Design review of the part shown in the three views and the two pictorial views. Dimensions are in mm from the part's minimum x, y and z. Coordinates: 2 decimals unless noted, no trailing zeros. Loops run counter-clockwise (first coordinate to the right, second up) from the corner with the lowest first, then second, coordinate; pieces in that order, holes last. Notation, with made-up numbers: M -34.75,12 L 20.25,12 A19 ccw 20.25,38 Z; hole C -1.75,79 d9. An arc over 180 degrees is marked long. Put each result on its own line as item: value. Start each with the question number.
(1) Take a section at D-D, the plane x = 14.25. Give the boundary of the cut face in (y, z), then the cut area to 3 significant figures.
(2) Take a section at B-B, the plane x = 2.5. Give the boundary of the cut face in (y, z).
(3) Take a section at C-C, the plane y = 0.95. Give the boundary of the cut face in (x, z), then the cut area to 3 significant figures.
(4) Clearance check with flat-ended pins moving along their axes: pin 1 (1.2 mm diameter, centred on y = 3, z = 9, fed in from +X); pin 2 (1.8 mm diameter, centred on x = 2.5, z = 2.25, fed in from +Y); pin 3 (1.5 mm diameter, centred on x = 11.5, z = 3.5, fed in from -Y); pin 4 (1.2 mm diameter, centred on x = 9, y = 3, fed in from -Z). State where each tip first meets the part, or that it passes through.
(5) Take a section at A-A, the plane z = 2.25. Give the boundary of the cut face in (x, y).
(6) The part is to be moulded in two halves that separate along X. For the marked faces 1, 2, 3 and 4, say which applies: +X half, -X half, draft (parallel to the pull), parting line (faces both ways), or undercut.
(7) For probe 1 along X at (y, z) = (0.95, 2.25); probe 2 along Y at (x, z) = (15, 3.75); probe 3 along Z at (x, y) = (2, 0.7), list the stretches that pass through material, from the lowest coordinate up. Write a range as [from, to].
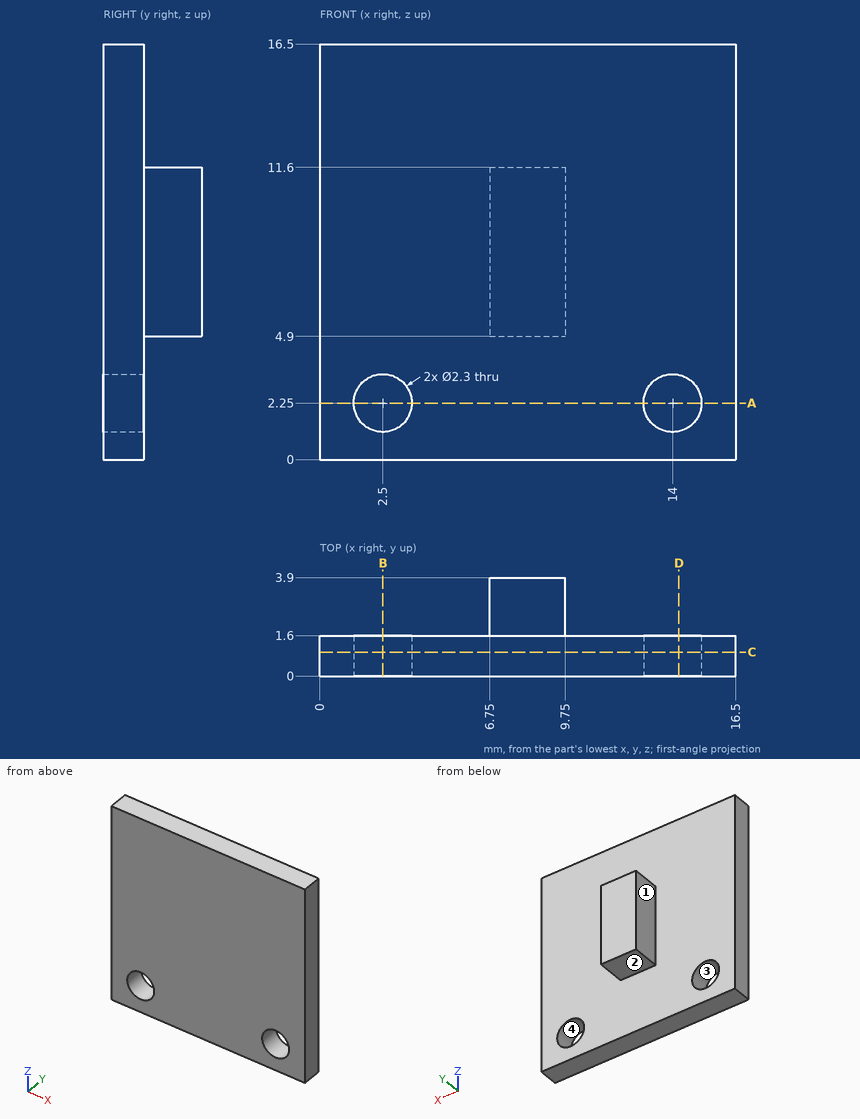
Computed values:
1. outline: M 0,0 L 1.6,0 L 1.6,1.13 L 0,1.13 Z; M 0,3.37 L 1.6,3.37 L 1.6,16.5 L 0,16.5 Z
1. area: 22.8 mm^2
2. outline: M 0,0 L 1.6,0 L 1.6,1.1 L 0,1.1 Z; M 0,3.4 L 1.6,3.4 L 1.6,16.5 L 0,16.5 Z
3. outline: M 0,0 L 16.5,0 L 16.5,16.5 L 0,16.5 Z; hole C 2.5,2.25 d2.3; hole C 14,2.25 d2.3
3. area: 264 mm^2
4. pin 1: stops at x = 9.75
4. pin 2: passes through
4. pin 3: stops at y = 0
4. pin 4: stops at z = 4.9
5. outline: M 0,0 L 1.35,0 L 1.35,1.6 L 0,1.6 Z; M 3.65,0 L 12.85,0 L 12.85,1.6 L 3.65,1.6 Z; M 15.15,0 L 16.5,0 L 16.5,1.6 L 15.15,1.6 Z
6. face 1: -X half
6. face 2: draft
6. face 3: undercut
6. face 4: undercut
7. probe 1: x = [0, 1.35], [3.65, 12.85], [15.15, 16.5]
7. probe 2: y = [0, 1.6]
7. probe 3: z = [0, 1.21], [3.29, 16.5]
